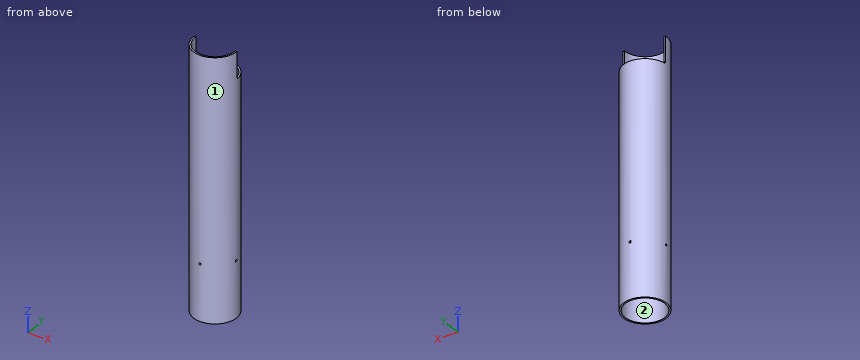
```python
from build123d import *

# Parameters (mm, degrees)
SKETCH_R             = 20
SKETCH_R_2           = 18.5
PAD_DEPTH            = 240
SKETCH001_R          = 1
POCKET_DEPTH         = 20.001
POCKET_DEPTH_BACK    = -20.001
SKETCH002_R          = 1
POCKET001_DEPTH      = 20.001
POCKET001_DEPTH_BACK = -20.001


with BuildPart() as part:
    # Sketch → Pad (new body)
    with BuildSketch(Plane.XY):
        Circle(SKETCH_R)
        Circle(SKETCH_R_2, mode=Mode.SUBTRACT)
    extrude(amount=PAD_DEPTH)

    # Sketch001 → Pocket (cut, two sides)
    with BuildSketch(Plane.YZ) as pocket_sk:
        with Locations((0, 52)):
            Circle(SKETCH001_R)
        with BuildLine():
            Line((1, 240), (23, 240))
            Line((23, 240), (23, 215))
            Line((23, 215), (3, 215))
            ThreePointArc((1, 217), (1.585786, 215.585786), (3, 215))
            Line((1, 217), (1, 240))
        make_face()
    extrude(amount=-POCKET_DEPTH, mode=Mode.SUBTRACT)
    extrude(pocket_sk.sketch, amount=-POCKET_DEPTH_BACK, mode=Mode.SUBTRACT)

    # Sketch002 → Pocket001 (cut, two sides)
    with BuildSketch(Plane.XZ) as pocket001_sk:
        with Locations((0, 52)):
            Circle(SKETCH002_R)
    extrude(amount=-POCKET001_DEPTH, mode=Mode.SUBTRACT)
    extrude(pocket001_sk.sketch, amount=-POCKET001_DEPTH_BACK, mode=Mode.SUBTRACT)


solid = part.part
```
Part model, mm, in its own coordinate system. Face numbers are marked on the shaded views. Give positions to 0.01 mm unless a question says otherwise; leave off trailing zeros. Write each loop counter-clockwise with the first axis right and the second up, starting at its lowest first coordinate (ties: lowest second). Pieces come first, ordered by that corner, then holes. Notation, with made-up numbers: M 43,48 L 57,48 A24 ccw 57,83 Z; hole C 77.5,54 d6. An arc over 180 degrees is marked long. Use CSV: the item, a comma, the result in double quotes.
Item 1: Pull direction X, two halves, no side cores. Call the marked faces 1 and 2: +X half, -X half, draft (parallel to the pull), parting line (faces both ways), or undercut.
Taken from the geometry:
face 1,"parting line"
face 2,"undercut"
Item 2: Pin check, flat tips, straight feed: P1, Ø1.2, axis at y = 0, z = 52, coming from the -X side; P2, Ø1.2, axis at x = 19, z = 224, coming from the +Y side; P3, Ø1, axis at x = 10, z = 200.5, coming from the +Y side; P4, Ø2, axis at x = -12, z = 180, coming from the +Y side. Stop position of each tip, or through.
Taken from the geometry:
P1,"passes through"
P2,"stops at y = 1"
P3,"stops at y = 17.6"
P4,"stops at y = 16.7"
Item 3: Slice it at A-A on y = 15. Write the cut outline in (x, z).
Taken from the geometry:
outline,"M -13.23,0 L -10.83,0 L -10.83,215 L -13.23,215 Z; M 10.83,0 L 13.23,0 L 13.23,215 L 10.83,215 Z"
Item 4: Drill centre lines: probe 1 along Y at (x, z) = (0, 189); probe 2 along X at (y, z) = (3, 90); probe 3 along Z at (x, y) = (19, 0). Where is each one in solid material? Low to high.
Taken from the geometry:
probe 1,"y = -20 to -18.5, 18.5 to 20"
probe 2,"x = -19.77 to -18.26, 18.26 to 19.77"
probe 3,"z = 0 to 51, 53 to 240"
Item 5: Slice it at C-C on z = 127. Write the cut outline in (x, y), plus the area to 3 significant figures.
Taken from the geometry:
outline,"C 0,0 d40; hole C 0,0 d37"
area,"181 mm²"
Item 6: Slice it at B-B on x = 6.5. Write the cut outline in (y, z), plus the area to 3 significant figures.
Taken from the geometry:
outline,"M -18.91,0 L -17.32,0 L -17.32,240 L -18.91,240 Z; M 17.32,0 L 18.91,0 L 18.91,215 L 17.32,215 Z"
area,"725 mm²"
